Build history of the part. All positions in model axes, mm. Round coordinates to 2 decimals unless told otherwise and drop trailing zeros. Use CSV: the item, a comma, the result in double quotes.
Autodesk Inventor part; units mm, degrees
ref_plane "YZ Plane" through (0, 0, 0) normal (1, 0, 0) x (0, 1, 0)
ref_plane "XZ Plane" through (0, 0, 0) normal (0, 1, 0) x (-1, 0, 0)
ref_plane "XY Plane" through (0, 0, 0) normal (0, 0, 1) x (1, 0, 0)
sketch "Sketch1" plane through (0, 0, 0) normal (0, 1, 0) x (-1, 0, 0)
  line L0 (0, -1.5) -> (0, -9.8)
  line L1 (0, -9.8) -> (1.1, -9.8)
  line L2 (1.1, -9.8) -> (1.1, -10.9)
  line L3 (1.1, -10.9) -> (2.2, -10.9)
  line L4 (2.2, -10.9) -> (2.2, -6.75)
  line L5 (0, -28.5) -> (0, -20.2)
  line L6 (0, -20.2) -> (1.1, -20.2)
  line L7 (1.1, -20.2) -> (1.1, -19.1)
  line L8 (1.1, -19.1) -> (2.2, -19.1)
  line L9 (2.2, -19.1) -> (2.2, -23.25)
  line L10 (1.5, 0) -> (9.8, 0)
  line L11 (9.8, 0) -> (9.8, -1.1)
  line L12 (9.8, -1.1) -> (10.9, -1.1)
  line L13 (10.9, -1.1) -> (10.9, -2.2)
  line L14 (10.9, -2.2) -> (6.75, -2.2)
  line L15 (28.5, 0) -> (20.2, 0)
  line L16 (20.2, 0) -> (20.2, -1.1)
  line L17 (20.2, -1.1) -> (19.1, -1.1)
  line L18 (19.1, -1.1) -> (19.1, -2.2)
  line L19 (19.1, -2.2) -> (23.25, -2.2)
  line L20 (30, -1.5) -> (30, -9.8)
  line L21 (30, -9.8) -> (28.9, -9.8)
  line L22 (28.9, -9.8) -> (28.9, -10.9)
  line L23 (28.9, -10.9) -> (27.8, -10.9)
  line L24 (27.8, -10.9) -> (27.8, -6.75)
  line L25 (30, -28.5) -> (30, -20.2)
  line L26 (30, -20.2) -> (28.9, -20.2)
  line L27 (28.9, -20.2) -> (28.9, -19.1)
  line L28 (28.9, -19.1) -> (27.8, -19.1)
  line L29 (27.8, -19.1) -> (27.8, -23.25)
  line L30 (28.5, -30) -> (20.2, -30)
  line L31 (20.2, -30) -> (20.2, -28.9)
  line L32 (20.2, -28.9) -> (19.1, -28.9)
  line L33 (19.1, -28.9) -> (19.1, -27.8)
  line L34 (19.1, -27.8) -> (23.25, -27.8)
  line L35 (1.5, -30) -> (9.8, -30)
  line L36 (9.8, -30) -> (9.8, -28.9)
  line L37 (9.8, -28.9) -> (10.9, -28.9)
  line L38 (10.9, -28.9) -> (10.9, -27.8)
  line L39 (10.9, -27.8) -> (6.75, -27.8)
  line L40 (6.75, -2.2) -> (6.75, -6.75)
  line L41 (6.75, -6.75) -> (2.2, -6.75)
  line L42 (2.2, -23.25) -> (6.75, -23.25)
  line L43 (6.75, -23.25) -> (6.75, -27.8)
  line L44 (23.25, -27.8) -> (23.25, -23.25)
  line L45 (23.25, -23.25) -> (27.8, -23.25)
  line L46 (27.8, -6.75) -> (23.25, -6.75)
  line L47 (23.25, -2.2) -> (23.25, -6.75)
  line L48 (9.2, -9.2) -> (20.8, -9.2)
  line L49 (20.8, -9.2) -> (20.8, -20.8)
  line L50 (20.8, -20.8) -> (9.2, -20.8)
  line L51 (9.2, -20.8) -> (9.2, -9.2)
  line L52 (23.25, -6.75) -> (23.25, -5.194)
  line L53 (23.25, -6.75) -> (24.806, -6.75)
  line L54 (6.75, -6.75) -> (5.194, -6.75)
  line L55 (6.75, -6.75) -> (6.75, -5.194)
  line L56 (6.75, -23.25) -> (5.194, -23.25)
  line L57 (6.75, -23.25) -> (6.75, -24.806)
  line L58 (23.25, -23.25) -> (23.25, -24.806)
  line L59 (23.25, -23.25) -> (24.806, -23.25)
  line L60 (5.194, -23.25) -> (23.25, -5.194)
  line L61 (24.806, -6.75) -> (6.75, -24.806)
  circle A0 centre (15, -15) radius 3.4
  arc A1 (1.5, 0) -> (0, -1.5) centre (1.5, -1.5) ccw
  arc A2 (0, -28.5) -> (1.5, -30) centre (1.5, -28.5) ccw
  arc A3 (28.5, -30) -> (30, -28.5) centre (28.5, -28.5) ccw
  arc A4 (30, -1.5) -> (28.5, 0) centre (28.5, -1.5) ccw
  line L62 (27.5, -1.5) -> (25.85, -1.5)
  line L63 (24.85, -2.5) -> (24.85, -4.15)
  line L64 (25.85, -5.15) -> (27.5, -5.15)
  line L65 (28.5, -4.15) -> (28.5, -2.5)
  line L66 (27.5, -24.85) -> (25.85, -24.85)
  line L67 (24.85, -25.85) -> (24.85, -27.5)
  line L68 (25.85, -28.5) -> (27.5, -28.5)
  line L69 (28.5, -27.5) -> (28.5, -25.85)
  line L70 (4.15, -24.85) -> (2.5, -24.85)
  line L71 (1.5, -25.85) -> (1.5, -27.5)
  line L72 (2.5, -28.5) -> (4.15, -28.5)
  line L73 (5.15, -27.5) -> (5.15, -25.85)
  line L74 (4.15, -1.5) -> (2.5, -1.5)
  line L75 (1.5, -2.5) -> (1.5, -4.15)
  line L76 (2.5, -5.15) -> (4.15, -5.15)
  line L77 (5.15, -4.15) -> (5.15, -2.5)
  arc A5 (27.5, -5.15) -> (28.5, -4.15) centre (27.5, -4.15) ccw
  arc A6 (28.5, -2.5) -> (27.5, -1.5) centre (27.5, -2.5) ccw
  arc A7 (25.85, -1.5) -> (24.85, -2.5) centre (25.85, -2.5) ccw
  arc A8 (24.85, -4.15) -> (25.85, -5.15) centre (25.85, -4.15) ccw
  arc A9 (5.15, -2.5) -> (4.15, -1.5) centre (4.15, -2.5) ccw
  arc A10 (1.5, -4.15) -> (2.5, -5.15) centre (2.5, -4.15) ccw
  arc A11 (4.15, -5.15) -> (5.15, -4.15) centre (4.15, -4.15) ccw
  arc A12 (2.5, -1.5) -> (1.5, -2.5) centre (2.5, -2.5) ccw
  arc A13 (2.5, -24.85) -> (1.5, -25.85) centre (2.5, -25.85) ccw
  arc A14 (5.15, -25.85) -> (4.15, -24.85) centre (4.15, -25.85) ccw
  arc A15 (4.15, -28.5) -> (5.15, -27.5) centre (4.15, -27.5) ccw
  arc A16 (1.5, -27.5) -> (2.5, -28.5) centre (2.5, -27.5) ccw
  arc A17 (25.85, -24.85) -> (24.85, -25.85) centre (25.85, -25.85) ccw
  arc A18 (28.5, -25.85) -> (27.5, -24.85) centre (27.5, -25.85) ccw
  arc A19 (27.5, -28.5) -> (28.5, -27.5) centre (27.5, -27.5) ccw
  arc A20 (24.85, -27.5) -> (25.85, -28.5) centre (25.85, -27.5) ccw
  line L78 (24.806, -23.25) -> (6.75, -5.194)
  line L79 (23.25, -24.806) -> (5.194, -6.75)
  point P0 (0, 0)
  point P1 (0, -30)
  point P2 (9.2, -15)
  point P3 (0, -15)
  point P4 (15, 0)
  point P5 (15, -9.2)
  dimension "d52" = 9.8
  dimension "d61" = 6.8
  dimension "d62" = 1.5
  dimension "d75" = 1.5
  dimension "d76" = 1.5
  dimension "d81" = 1
  dimension "d82" = 1.556
  dimension "d83" = 1.556
  dimension "d84" = 1.556
  dimension "d85" = 1.556
  dimension "d86" = 1.556
  dimension "d87" = 1.556
  dimension "d88" = 1.556
extrude "Extrusion1" add sketch "Sketch1" along normal blind 500 contours A1 L10 L11 L12 L13 L14 L40 L41 L4 L3 L2 L1 L0 | L41 L40 L78 L48 L51 L79 | L79 A0 L60 L51 | L51 L48 L78 A0 L79 | L60 A0 L61 L50 L51 | L51 L50 L61 L43 L42 L60 | A0 L78 L60 L79 | L48 L60 A0 L78 | L42 L43 L39 L38 L37 L36 L35 A2 L5 L6 L7 L8 L9 | L60 L79 L61 A0 | L60 L78 L61 L79 | L60 L47 L46 L61 L49 L48 | L48 L49 L61 A0 L60 | L61 A0 L79 L50 | A0 L61 L78 L60 | L61 L78 A0 L79 | L47 L19 L18 L17 L16 L15 A4 L20 L21 L22 L23 L24 L46 | L79 A0 L78 L49 L50 | L50 L49 L78 L45 L44 L79 | L61 L49 L78 A0 | L44 L45 L29 L28 L27 L26 L25 A3 L30 L31 L32 L33 L34
sketch "Sketch2" plane through (0, 0, 0) normal (0, -1, 0) x (1, 0, 0)
  circle A0 centre (-15, -15) radius 3.5
  line L0 (-20.2, -30) -> (-9.8, -30)
  line L1 (-1.5, -30) -> (-9.8, -30)
  line L2 (-30, -9.8) -> (-30, -20.2)
  point P0 (0, 0)
  point P1 (-30, -15)
  point P2 (-15, -30)
  dimension "d91" = 7
extrude "Extrusion2" cut sketch "Sketch2" against normal blind 500
sketch "Sketch3" plane through (0, 0, 0) normal (0, -1, 0) x (1, 0, 0)
  point P0 (0, 0)
sketch "Sketch4" plane through (-19.244, 0, -9.2) normal (0, 0, 1) x (1, 0, 0)
  point P0 (34.244, 485)
sketch "Sketch5" plane through (-19.244, 0, -9.2) normal (0, 0, 1) x (1, 0, 0)
  point P0 (-25.756, 15)
properties part number "Balka"
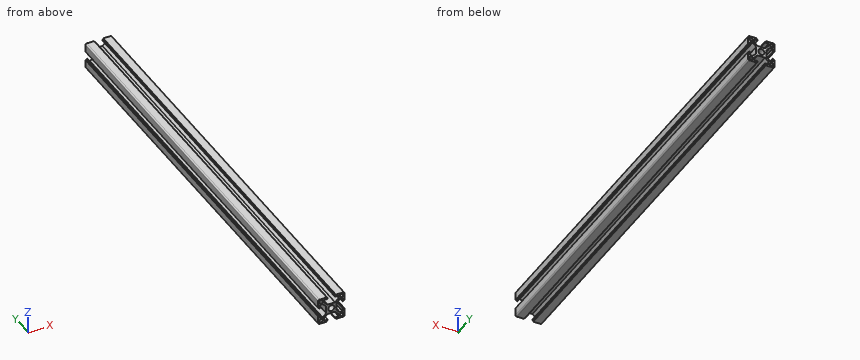
(1) Cut at A-A, the plane y = 368.5. Count the separate pieces of the cut face and the enclosed holes in it, and give its area (3 significant figures).
Answer block:
separate pieces,"1"
enclosed holes,"5"
area,"330 mm²"
(2) Drop flat-ended pins along their axis: pin 1 (3 mm diameter, centred on x = -15, y = 123, fed in from +Z); pin 2 (2 mm diameter, centred on x = -12, y = 266.5, fed in from -Z); pin 3 (5 mm diameter, centred on x = -24.5, z = -18, fed in from +Y). Give the stop position or say it passes through.
Answer block:
pin 1,"stops at z = -9.2"
pin 2,"stops at z = -20.8"
pin 3,"passes through"
(3) Wall check: line 1 (X direction, y = 414.5, z = -26.5); line 2 (Z direction, x = -15, y = 289.5). Give the ranges that are in metal, low to high. Write a range as from..to.
Answer block:
line 1,"x = -30..-28.5, -24.85..-23.25, -6.75..-5.15, -1.5..0"
line 2,"z = -20.8..-18.5, -11.5..-9.2"
